For this review, take the finished solid that the model builds, in its own axes (mm). A direction names the side the tool comes from. Give positions to 0.01 mm unless a question says otherwise; leave off trailing zeros. Loops run counter-clockwise (first coordinate to the right, second up) from the corner with the lowest first, then second, coordinate; pieces in that order, holes last. Notation, with made-up numbers: (89, 62) - (108, 62) arc R22 cw to (108, 83) - close; hole circle Ø2 at (-22, -21.75). An arc over 180 degrees is marked (long way). Answer in a Markdown table with one row per item.
```python
from build123d import *

# Parameters (mm, degrees)
SKETCH_1_W          = 110
SKETCH_1_H          = 20
SKETCH_1_R          = 1.7
EXTRUDE_1_DEPTH     = 4.5
SKETCH_2_W          = 20
SKETCH_2_H          = 8
EXTRUDE_2_DEPTH     = 45
CUT_EXTRUDE_1_DEPTH = 1.3
SKETCH_4_W          = 10
SKETCH_4_H          = 10
EXTRUDE_3_DEPTH     = 4.5
SKETCH_5_R          = 1.9
CUT_EXTRUDE_2_DEPTH = 77.155752448
CUT_EXTRUDE_3_DEPTH = 2.6
SKETCH_7_R          = 1.7
CUT_EXTRUDE_4_DEPTH = 79.898343651
CUT_EXTRUDE_5_DEPTH = 1.3
FILLET_1_R          = 2


with BuildPart() as part:
    # 草图1 → 凸台-拉伸1 (new body)
    with BuildSketch(Plane.XY):
        with Locations((0, 10)):
            Rectangle(SKETCH_1_W, SKETCH_1_H)
        with Locations((-45, 14)):
            Circle(SKETCH_1_R, mode=Mode.SUBTRACT)
        with Locations((-30, 14)):
            Circle(SKETCH_1_R, mode=Mode.SUBTRACT)
        with Locations((-15, 14)):
            Circle(SKETCH_1_R, mode=Mode.SUBTRACT)
        with Locations((15, 14)):
            Circle(SKETCH_1_R, mode=Mode.SUBTRACT)
        with Locations((30, 14)):
            Circle(SKETCH_1_R, mode=Mode.SUBTRACT)
        with Locations((45, 14)):
            Circle(SKETCH_1_R, mode=Mode.SUBTRACT)
    extrude(amount=EXTRUDE_1_DEPTH)

    # 草图2 → 凸台-拉伸2 (add)
    with BuildSketch(Plane.XY.offset(4.5)):
        with Locations((-45, 4)):
            Rectangle(SKETCH_2_W, SKETCH_2_H)
        with Locations((45, 4)):
            Rectangle(SKETCH_2_W, SKETCH_2_H)
    extrude(amount=EXTRUDE_2_DEPTH)

    # 草图3 → 切除-拉伸1 (cut)
    with BuildSketch(Plane.XY.offset(4.5)):
        Polygon((-45, 17.22), (-47.7886018, 15.61), (-47.7886018, 12.39), (-45, 10.78), (-42.2113982, 12.39), (-42.2113982, 15.61), align=None)
        Polygon((-30, 17.22), (-32.7886018, 15.61), (-32.7886018, 12.39), (-30, 10.78), (-27.2113982, 12.39), (-27.2113982, 15.61), align=None)
        Polygon((-15, 17.22), (-17.7886018, 15.61), (-17.7886018, 12.39), (-15, 10.78), (-12.2113982, 12.39), (-12.2113982, 15.61), align=None)
        Polygon((15, 17.22), (12.2113982, 15.61), (12.2113982, 12.39), (15, 10.78), (17.7886018, 12.39), (17.7886018, 15.61), align=None)
        Polygon((30, 17.22), (27.2113982, 15.61), (27.2113982, 12.39), (30, 10.78), (32.7886018, 12.39), (32.7886018, 15.61), align=None)
        Polygon((45, 17.22), (42.2113982, 15.61), (42.2113982, 12.39), (45, 10.78), (47.7886018, 12.39), (47.7886018, 15.61), align=None)
    extrude(amount=-CUT_EXTRUDE_1_DEPTH, mode=Mode.SUBTRACT)

    # 草图4 → 凸台-拉伸3 (add)
    with BuildSketch(Plane.XY.offset(4.5)):
        with Locations((19.238259457, 22.3806251)):
            Rectangle(SKETCH_4_W, SKETCH_4_H)
        with Locations((-31.561740543, 22.3806251)):
            Rectangle(SKETCH_4_W, SKETCH_4_H)
    extrude(amount=-EXTRUDE_3_DEPTH)

    # 草图5 → 切除-拉伸2 (cut, through all)
    with BuildSketch(Plane.XY.offset(4.5)):
        with Locations((19.238259457, 22.3806251)):
            Circle(SKETCH_5_R)
        with Locations((-31.561740543, 22.3806251)):
            Circle(SKETCH_5_R)
    extrude(amount=-CUT_EXTRUDE_2_DEPTH, mode=Mode.SUBTRACT)

    # 草图6 → 切除-拉伸3 (cut)
    with BuildSketch(Plane(origin=(0, 0, 0), x_dir=(-1, 0, 0), z_dir=(0, 0, -1))):
        Polygon((34.861740543, 22.3806251), (33.211740543, 25.238508932), (29.911740543, 25.238508932), (28.261740543, 22.3806251), (29.911740543, 19.522741267), (33.211740543, 19.522741267), align=None)
        Polygon((-15.938259457, 22.3806251), (-17.588259457, 25.238508932), (-20.888259457, 25.238508932), (-22.538259457, 22.3806251), (-20.888259457, 19.522741267), (-17.588259457, 19.522741267), align=None)
    extrude(amount=-CUT_EXTRUDE_3_DEPTH, mode=Mode.SUBTRACT)

    # 草图7 → 切除-拉伸4 (cut, through all)
    with BuildSketch(Plane.XZ):
        with Locations(Location((-51, 43.5, 0), (0, 0, 270))):
            Circle(SKETCH_7_R)
        with Locations(Location((-39, 43.5, 0), (0, 0, 270))):
            Circle(SKETCH_7_R)
        with Locations(Location((-45, 33.5, 0), (0, 0, 270))):
            Circle(SKETCH_7_R)
        with Locations(Location((39, 43.5, 0), (0, 0, 270))):
            Circle(SKETCH_7_R)
        with Locations(Location((51, 43.5, 0), (0, 0, 270))):
            Circle(SKETCH_7_R)
        with Locations(Location((45, 33.5, 0), (0, 0, 270))):
            Circle(SKETCH_7_R)
    extrude(amount=-CUT_EXTRUDE_4_DEPTH, mode=Mode.SUBTRACT)

    # 草图8 → 切除-拉伸5 (cut)
    with BuildSketch(Plane(origin=(0, 8, 0), x_dir=(1, 0, 0), z_dir=(0, 1, 0))):
        Polygon((51, -46.72), (53.7886018, -45.11), (53.7886018, -41.89), (51, -40.28), (48.2113982, -41.89), (48.2113982, -45.11), align=None)
        Polygon((39, -46.72), (41.7886018, -45.11), (41.7886018, -41.89), (39, -40.28), (36.2113982, -41.89), (36.2113982, -45.11), align=None)
        Polygon((45, -36.72), (47.7886018, -35.11), (47.7886018, -31.89), (45, -30.28), (42.2113982, -31.89), (42.2113982, -35.11), align=None)
        Polygon((-39, -46.72), (-36.2113982, -45.11), (-36.2113982, -41.89), (-39, -40.28), (-41.7886018, -41.89), (-41.7886018, -45.11), align=None)
        Polygon((-51, -46.72), (-48.2113982, -45.11), (-48.2113982, -41.89), (-51, -40.28), (-53.7886018, -41.89), (-53.7886018, -45.11), align=None)
        Polygon((-45, -36.72), (-42.2113982, -35.11), (-42.2113982, -31.89), (-45, -30.28), (-47.7886018, -31.89), (-47.7886018, -35.11), align=None)
    extrude(amount=-CUT_EXTRUDE_5_DEPTH, mode=Mode.SUBTRACT)

    # 圆角1
    fillet_1_edges = [part.edges().sort_by_distance(p)[0] for p in [
        (24.238259457, 20, 2.25),
        (14.238259457, 20, 2.25),
        (24.238259457, 27.3806251, 2.25),
        (14.238259457, 27.3806251, 2.25),
        (-26.561740543, 27.3806251, 2.25),
        (-36.561740543, 20, 2.25),
        (-36.561740543, 27.3806251, 2.25),
        (-26.561740543, 20, 2.25),
        (-35, 4, 4.5),
        (-45, 8, 4.5),
        (-55, 4, 49.5),
        (-35, 4, 49.5),
        (45, 8, 4.5),
        (35, 4, 4.5),
        (55, 4, 49.5),
        (35, 4, 49.5),
        (-55, 20, 2.25),
        (55, 20, 2.25),
    ]]
    fillet(fillet_1_edges, radius=FILLET_1_R)


solid = part.part
```
1. Clearance check with flat-ended pins moving along their axes: pin 1 (6 mm diameter, centred on x = 48.5, z = 27, fed in from +Y); pin 2 (4.5 mm diameter, centred on x = -39, z = 43.5, fed in from +Y); pin 3 (5 mm diameter, centred on x = 12, y = 9.5, fed in from +Z); pin 4 (4 mm diameter, centred on x = -45, y = 14, fed in from -Z). State where each tip first meets the part, or that it passes through.
Values:
| item | result |
|---|---|
| pin 1 | stops at y = 8 |
| pin 2 | stops at y = 6.7 |
| pin 3 | stops at z = 4.5 |
| pin 4 | stops at z = 0 |
2. Wall thickness on line 1 (X direction, y = 4, z = 43.5); line 2 (Y direction, x = -15, z = 0.7); line 3 (X direction, y = 5.75, z = 28.5): over which ranges is each line inside the solid? List them lowest first. Write a range as [from, to].
Values:
| item | result |
|---|---|
| line 1 | x = [-55, -52.7], [-49.3, -40.7], [-37.3, -35], [35, 37.3], [40.7, 49.3], [52.7, 55] |
| line 2 | y = [0, 12.3], [15.7, 20] |
| line 3 | x = [-55, -35], [35, 55] |
3. For faces 5 (the face through (-34.4, 3.96, 5.07)), 6 (the face through (-40.3, 6.7, 44.9)), 7 (the face through (-46.3, 12.6, 3.2)), 8 (the face through (16.775, 20.932, 1.282)), list the 3-axis set-ups (+Z, -Z, +X, -X, +Y, -Y) from which the entire face can be reached by the end or side of a thin tool; tool diameter is ignored.
Values:
| item | result |
|---|---|
| face 5 | +Z, +Y, -Y |
| face 6 | +Y |
| face 7 | +Z |
| face 8 | -Z |
4. We need section A-A, the plane z = 13. Give the boundary of the cut face in (x, y).
Values:
| item | result |
|---|---|
| outline | (-55, 0) - (-35, 0) - (-35, 8) - (-55, 8) - close; (35, 0) - (55, 0) - (55, 8) - (35, 8) - close |
5. Mouldability with a two-part tool opening along Y and no side actions: class faces 1 (the face through (-34.025, 20.932, 1.282)), 2 (the face through (-33.46, 22.46, 3.56)), 3 (the face through (34.4, 3.96, 5.07)), 4 (the face through (14.81, 26.78, 2.22)) as released by +Y, released by -Y, zero draft, split by the parting line, or undercut.
Values:
| item | result |
|---|---|
| face 1 | undercut |
| face 2 | undercut |
| face 3 | zero draft |
| face 4 | released by +Y |
